Geometry check sheet. Reference: the model listing, model coordinates, mm. A direction names the side the tool comes from. Coordinates: 2 decimals unless noted, no trailing zeros. Write each loop counter-clockwise with the first axis right and the second up, starting at its lowest first coordinate (ties: lowest second). Pieces come first, ordered by that corner, then holes. Notation, with made-up numbers: M 43.5,56.25 L 74.5,56.25 A13 cw 74.5,68.25 Z; hole C -23.75,-16.75 d8. An arc over 180 degrees is marked long. Write each question's results on one line, items separated by ' | '.
```python
from build123d import *

# Parameters (mm, degrees)
F1_DEPTH = 5


with BuildPart() as f1:
    # F0 (on Front) → F1 (new body)
    with BuildSketch(Plane.XZ):
        with BuildLine():
            ThreePointArc((-32.5, 0), (0, 32.5), (32.5, 0))
            Line((32.5, 0), (42.5, 0))
            ThreePointArc((42.5, 0), (46.035534, 1.464466), (47.5, 5))
            Line((47.5, 5), (47.5, 30))
            ThreePointArc((47.5, 30), (43.106602, 40.606602), (32.5, 45))
            Line((32.5, 45), (-67.5, 45))
            Line((-67.5, 45), (-67.5, 40))
            Line((-67.5, 40), (-82.5, 40))
            Line((-82.5, 40), (-82.5, 45))
            Line((-82.5, 45), (-125, 45))
            ThreePointArc((-125, 45), (-135.606602, 40.606602), (-140, 30))
            Line((-140, 30), (-140, 0))
            Line((-140, 0), (-130, 0))
            Line((-130, 0), (-32.5, 0))
        make_face()
    extrude(amount=F1_DEPTH)


solid = f1.part
```
Q1. Sectioned sample at D-D on z = 37. Record the cut outline in (x, y).
Geometry check:
outline: M -138.27,-5 L 45.77,-5 L 45.77,0 L -138.27,0 Z
Q2. Sectioned sample at C-C on x = 0. Record the cut outline in (y, z), and give its area (3 significant figures).
Geometry check:
outline: M -5,32.5 L 0,32.5 L 0,45 L -5,45 Z | area: 62.5 mm2
Q3. Depth check by flat-ended pin: P1, Ø1, axis at x = 27.5, y = -3, coming from the -Z side; P2, Ø1.5, axis at x = -77, y = -3.5, coming from the +Z side; P3, Ø12, axis at x = 2, z = 23, coming from the -Y side. Enter the tip coordinate at first touch or a pass-through.
Geometry check:
P1: stops at z = 16.5 | P2: stops at z = 40 | P3: passes through
Q4. Sectioned sample at A-A on z = 13. Record the cut outline in (x, y).
Geometry check:
outline: M -140,-5 L -29.79,-5 L -29.79,0 L -140,0 Z; M 29.79,-5 L 47.5,-5 L 47.5,0 L 29.79,0 Z
Q5. Sectioned sample at B-B on y = -3.1. Record the cut outline in (x, z), and give its area (3 significant figures).
Geometry check:
outline: M -140,0 L -32.5,0 A32.5 cw 32.5,0 L 42.5,0 A5 ccw 47.5,5 L 47.5,30 A15 ccw 32.5,45 L -67.5,45 L -67.5,40 L -82.5,40 L -82.5,45 L -125,45 A15 ccw -140,30 Z | area: 6,600 mm2
Q6. Access from +Z, -Z, +X, -X, +Y, -Y to the whole of each face (thin tool, end or side, straight path). Record for faces 4 (the flat face through (-75, -2, 40)), 5 (the cylindrical face through (-0.715, -2.465, 32.492)).
Geometry check:
face 4: +Z, +Y, -Y | face 5: -Z, +Y, -Y
Q7. Mould release check, pull along X, two halves, no side actions. Record for faces 1 (the flat face through (-68, 0, 23)), 2 (the cylindrical face through (46, -2.46, 1.43)), 3 (the flat face through (-67.5, -2, 43)): pulls with the +X half, pulls with the -X half, needs draft (parallel to the pull), parting line crosses it, or undercut.
Geometry check:
face 1: needs draft | face 2: pulls with the +X half | face 3: undercut
Q8. Scan lines: probe 1 along Z at (x, y) = (33.5, -2.45); probe 2 along X at (y, z) = (-4.05, 13.5); probe 3 along X at (y, z) = (-1.45, 26). Record each from-to range of solid material in increasing order.
Geometry check:
probe 1: z = 0 to 44.97 | probe 2: x = -140 to -29.56, 29.56 to 47.5 | probe 3: x = -140 to -19.5, 19.5 to 47.5
